```python
from build123d import *

# Parameters (mm, degrees)
CROQUIS1_W                 = 86
CROQUIS1_H                 = 10.691540382
CROQUIS1_W_2               = 12
CROQUIS1_H_2               = 13.591389859
CROQUIS2_R                 = 3
CORTAR_EXTRUIR1_DEPTH      = 14.591389858
CORTAR_EXTRUIR1_DEPTH_BACK = 14.591389858


with BuildPart() as part:
    # Croquis1 → Revolución3 (revolve)
    with BuildSketch(Plane.XY):
        with Locations((43, -5.345770191)):
            Rectangle(CROQUIS1_W, CROQUIS1_H)
        Polygon((0, -10.691540382), (0, 0), (-4, -4), (-4, -10.691540382), align=None)
        with Locations((96, -3.895845453)):
            Rectangle(CROQUIS1_W_2, CROQUIS1_H_2)
        Polygon((90, 2.899849477), (86, 0), (86, -10.691540382), (90, -10.691540382), align=None)
        Polygon((106, 0), (102, 2.899849477), (102, -10.691540382), (106, -10.691540382), align=None)
    revolve(axis=Axis((-4, -10.691540382, 0), (1, 0, 0)))

    # Croquis2 → Cortar-Extruir1 (cut, two sides)
    with BuildSketch(Plane.XY) as cortar_extruir1_sk:
        with Locations((11, -10.691540382)):
            Circle(CROQUIS2_R)
    extrude(amount=CORTAR_EXTRUIR1_DEPTH, mode=Mode.SUBTRACT)
    extrude(cortar_extruir1_sk.sketch, amount=-CORTAR_EXTRUIR1_DEPTH_BACK, mode=Mode.SUBTRACT)


solid = part.part
```
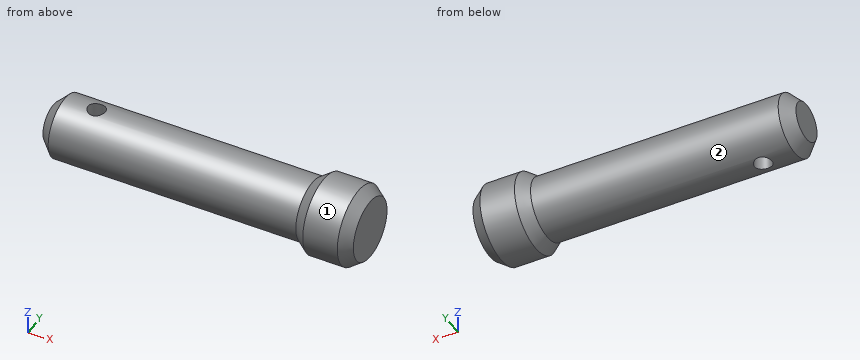
Design review of the part built by this model. Coordinates are the model's own, in mm. Face numbers are marked on the shaded views. A direction names the side the tool comes from. Coordinates: 2 decimals unless noted, no trailing zeros. Loops run counter-clockwise (first coordinate to the right, second up) from the corner with the lowest first, then second, coordinate; pieces in that order, holes last. Notation, with made-up numbers: (10.25, 0) -> (42.25, 0) arc R19 ccw to (42.25, 16) -> close; hole circle Ø7 at (30.5, 7.5). An arc over 180 degrees is marked (long way). Answer as a JSON object with one key per item and string values.
Q1. Take a section at A-A on z = 0. Give the boundary of the cut face in (x, y), plus the area to 3 significant figures.
Answer block:
{"outline": "(-4, -17.38) -> (0, -21.38) -> (86, -21.38) -> (90, -24.28) -> (102, -24.28) -> (106, -21.38) -> (106, 0) -> (102, 2.9) -> (90, 2.9) -> (86, 0) -> (0, 0) -> (-4, -4) -> close; hole circle Ø6 at (11, -10.69)", "area": "2,400 mm^2"}
Q2. Take a section at B-B on x = 98.5. Give the boundary of the cut face in (y, z), plus the area to 3 significant figures.
Answer block:
{"outline": "circle Ø27.18 at (-10.69, 0)", "area": "580 mm^2"}
Q3. Take a section at C-C on x = 11. Give the boundary of the cut face in (y, z).
Answer block:
{"outline": "(-13.69, -10.26) -> (-13.69, 10.26) arc R10.69 ccw to start; (-7.69, -10.26) arc R10.69 ccw to (-7.69, 10.26) -> close"}
Q4. Clearance check with flat-ended pins moving along their axes: pin 1 Ø6 at (x, z) = (83, 8.5) entering from -Y; pin 2 Ø1.5 at (x, y) = (42.5, -1) entering from -Z; pin 3 Ø5 at (x, y) = (57.5, -5) entering from -Z. State where each tip first meets the part, or that it passes through.
Answer block:
{"pin 1": "stops at y = -19.86", "pin 2": "stops at z = -5.86", "pin 3": "stops at z = -10.2"}
Q5. Tool access review of the marked faces 1 and 2: name each direction out of +Z, -Z, +X, -X, +Y, -Y from which nothing blocks a thin tool from reaching the whole face with its end or side.
Answer block:
{"face 1": "+X, -X", "face 2": "-X"}
Q6. To check wall thickness, follow L1, parallel to Y at x = 11, z = -0.5; L2, parallel to X at y = -10.75, z = -0.25; L3, parallel to X at y = -9.5, z = 5. State the ranges of each line that lie inside material, in increasing order.
Answer block:
{"L1": "y = -21.37 to -13.69, -7.69 to -0.01", "L2": "x = -4 to 8, 14 to 106", "L3": "x = -4 to 8.25, 13.75 to 106"}
